Print and shaded views of the part. All mm, measured from the part's lowest x, y and z. A direction names the side the tool comes from. Give positions to 0.01 mm unless a question says otherwise; leave off trailing zeros. Loops run counter-clockwise (first coordinate to the right, second up) from the corner with the lowest first, then second, coordinate; pieces in that order, holes last. Notation, with made-up numbers: (33, 54) -> (92, 54) arc R32 cw to (92, 87) -> close; hole circle Ø3 at (30.25, 19). An arc over 180 degrees is marked (long way). Write each question's results on one line, items separated by ' | '. Start each with the question number.
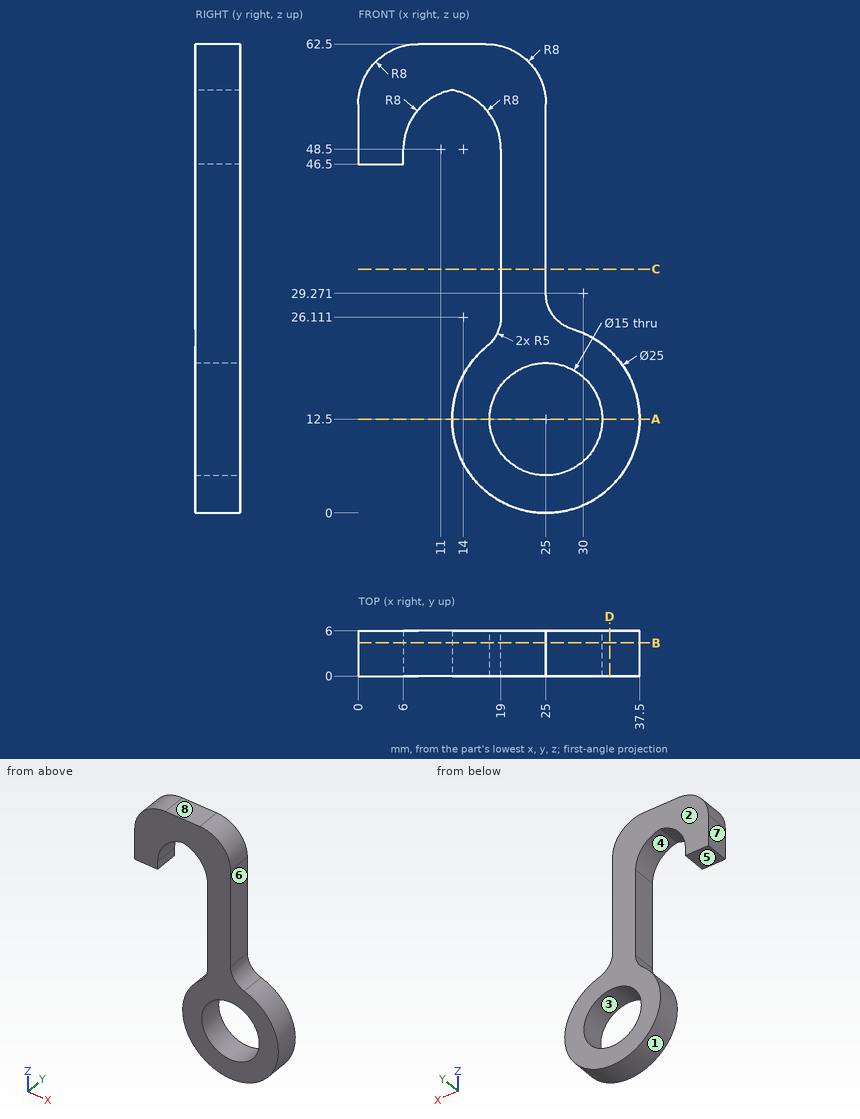
Q1. Drop flat-ended pins along their axis: pin 1 (3 mm diameter, centred on y = 3, z = 43.5, fed in from +X); pin 2 (5 mm diameter, centred on x = 26.5, z = 6.5, fed in from -Y); pin 3 (5 mm diameter, centred on x = 14.5, z = 36, fed in from +Y); pin 4 (3 mm diameter, centred on x = 1.5, y = 4, fed in from -Z). Give the stop position or say it passes through.
Q2. Mould opens along X. For the marked faces 1, 2 and 3 say: pulls with the +X half, pulls with the -X half, needs draft (parallel to the pull), parting line crosses it, or undercut.
Q3. Saw through at D-D, the plane x = 33.5. List the corners of the cut face in (y, z) (1 decimal).
Q4. Saw through at C-C, the plane z = 32.5. List the corners of the cut face in (x, y), then the cut area to 3 significant figures.
Q5. Saw through at A-A, the plane z = 12.5. List the corners of the cut face in (x, y).
Q6. Which spindle directions (+Z, -Z, +X, -X, +Y, -Y) get a long thin tool onto all of the face, cutting with end or side? Do the marked faces 4, 5, 6, 7 and 8. Say none if no direction does.
Q7. Wall check: L1, parallel to X at y = 3.05, z = 52.5; L2, parallel to X at y = 1.05, z = 30; L3, parallel to X at y = 1.25, z = 11. Give the ranges that are in metal, low to high.
Q8. Saw through at B-B, the plane y = 4.4. List the corners of the cut face in (x, z), then the cut area to 3 significant figures.
Answer block:
1) pin 1: stops at x = 25 | pin 2: stops at y = 0 | pin 3: passes through | pin 4: stops at z = 46.5
2) face 1: parting line crosses it | face 2: needs draft | face 3: undercut
3) outline: (0, 3.3) -> (6, 3.3) -> (6, 21.7) -> (0, 21.7) -> close
4) outline: (19, 0) -> (25, 0) -> (25, 6) -> (19, 6) -> close | area: 36.0 mm2
5) outline: (12.5, 0) -> (17.5, 0) -> (17.5, 6) -> (12.5, 6) -> close; (32.5, 0) -> (37.5, 0) -> (37.5, 6) -> (32.5, 6) -> close
6) face 4: +Y, -Y | face 5: -Z, -X, +Y, -Y | face 6: +Z, +X, +Y, -Y | face 7: +Z, -Z, -X, +Y, -Y | face 8: +Z, +X, -X, +Y, -Y
7) L1: x = 0 to 7.07, 17.93 to 25 | L2: x = 19 to 25 | L3: x = 12.59 to 17.65, 32.35 to 37.41
8) outline: (0, 46.5) -> (6, 46.5) -> (6, 48.5) arc R8 cw to (12.5, 56.36) arc R8 cw to (19, 48.5) -> (19, 26.11) arc R5 cw to (17.14, 22.22) arc R12.5 ccw (long way) to (28.57, 24.48) arc R5 cw to (25, 29.27) -> (25, 54.5) arc R8 ccw to (17, 62.5) -> (8, 62.5) arc R8 ccw to (0, 54.5) -> close; hole circle Ø15 at (25, 12.5) | area: 720 mm2
